Could you check a few things on this drawing? It's one solid part, dimensions in mm from its lowest x, y, z. A direction names the side the tool comes from. Round coordinates to 2 decimals unless told otherwise and drop trailing zeros. Write each loop counter-clockwise with the first axis right and the second up, starting at its lowest first coordinate (ties: lowest second). Pieces come first, ordered by that corner, then holes. Notation, with made-up numbers: (22, 29.5) -> (40, 29.5) arc R30 cw to (40, 60.5) -> close; hole circle Ø11 at (-12.5, 84.25). An arc over 180 degrees is marked (long way). Answer as CSV lines item,"result".
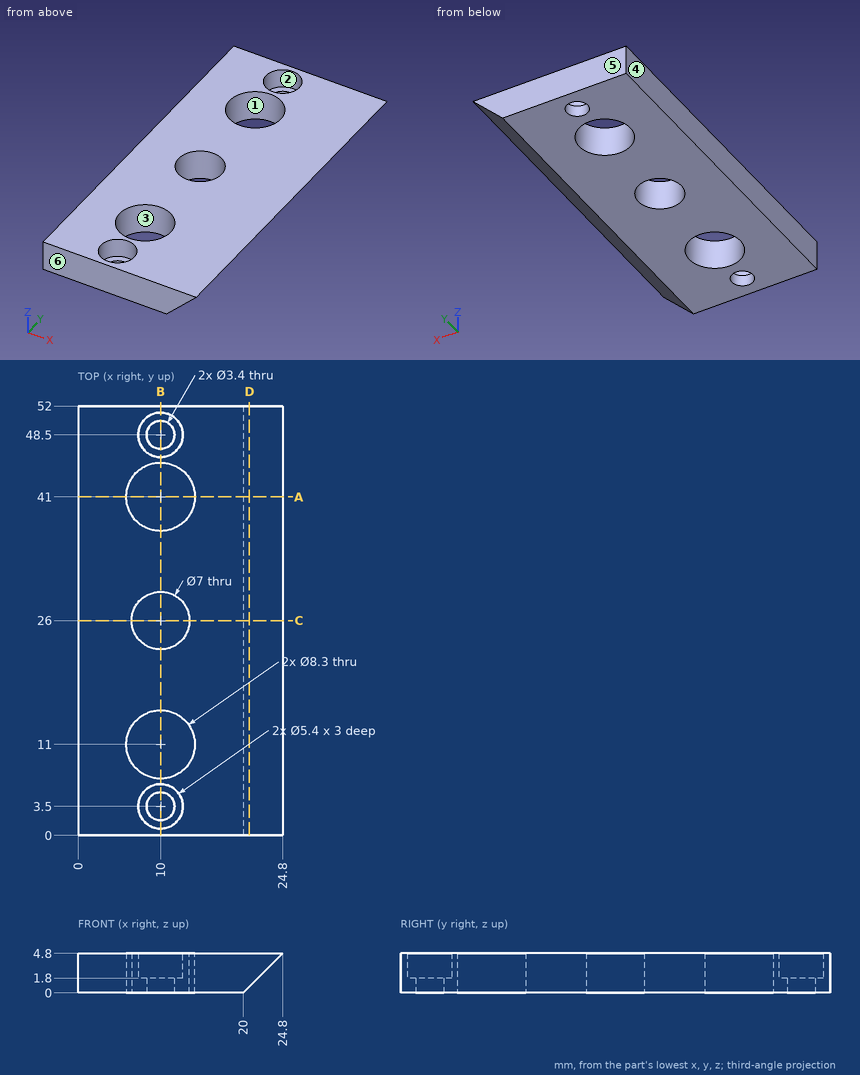
1. If we mould it in two halves opening along Y, with no side actions, what happens to the marked faces 3, 4, 5 and 6? For each: released by +Y, released by -Y, zero draft, split by the parting line, or undercut.
Numbers:
face 3,"undercut"
face 4,"zero draft"
face 5,"released by +Y"
face 6,"released by -Y"
2. Suppose I cut it at D-D on x = 20.75. Please give me the cut outline in (y, z).
Numbers:
outline,"(0, 0.75) -> (52, 0.75) -> (52, 4.8) -> (0, 4.8) -> close"
3. Suppose I cut it at B-B on x = 10. Count the separate pieces of the cut face and the enclosed holes in it, and give its area (3 significant figures).
Numbers:
separate pieces,"6"
enclosed holes,"0"
area,"91.7 mm^2"
4. Suppose I cut it at A-A on y = 41. Please give me the cut outline in (x, z).
Numbers:
outline,"(0, 0) -> (5.85, 0) -> (5.85, 4.8) -> (0, 4.8) -> close; (14.15, 0) -> (20, 0) -> (24.8, 4.8) -> (14.15, 4.8) -> close"
5. For pin 1 Ø1.6 at (x, y) = (10, 48) entering from +Z; pin 2 Ø2.5 at (x, y) = (9.5, 4.5) entering from +Z; pin 3 Ø1 at (y, z) = (36.5, 1) entering from +X, each with a flat end and sliding along its axis, tell me the tip position at first contact or that it passes through.
Numbers:
pin 1,"passes through"
pin 2,"stops at z = 1.8"
pin 3,"stops at x = 21.5"
6. On a 3-axis mill with a long thin cutter (end or side, diameter ignored), from which of +Z, -Z, +X, -X, +Y, -Y can I reach the whole of each face in a straight line? I mean the marked faces 1 and 2. Say none if no direction works.
Numbers:
face 1,"+Z, -Z"
face 2,"+Z"
7. Suppose I cut it at C-C on y = 26. Please give me the cut outline in (x, z).
Numbers:
outline,"(0, 0) -> (6.5, 0) -> (6.5, 4.8) -> (0, 4.8) -> close; (13.5, 0) -> (20, 0) -> (24.8, 4.8) -> (13.5, 4.8) -> close"
8. If I drill on line 1 (Y direction, x = 10, z = 0.5); line 2 (Y direction, x = 10, z = 2.8); line 3 (X direction, y = 28, z = 4), over which ranges is the centre line in solid material (lowest first)?
Numbers:
line 1,"y = 0 to 1.8, 5.2 to 6.85, 15.15 to 22.5, 29.5 to 36.85, 45.15 to 46.8, 50.2 to 52"
line 2,"y = 0 to 0.8, 6.2 to 6.85, 15.15 to 22.5, 29.5 to 36.85, 45.15 to 45.8, 51.2 to 52"
line 3,"x = 0 to 7.13, 12.87 to 24"
